The figure shows three views and two pictorial views of one solid part (mm, origin at its lowest corner). Answer the questions. A direction names the side the tool comes from. Give positions to 0.01 mm unless a question says otherwise; leave off trailing zeros. Write each loop counter-clockwise with the first axis right and the second up, starting at its lowest first coordinate (ties: lowest second). Pieces come first, ordered by that corner, then holes. Notation, with made-up numbers: M 36.5,7.25 L 87.5,7.25 A18 cw 87.5,22.25 Z; hole C 41,-24.5 d10. An arc over 180 degrees is marked long. Return JSON: item names as keys, results as strings.
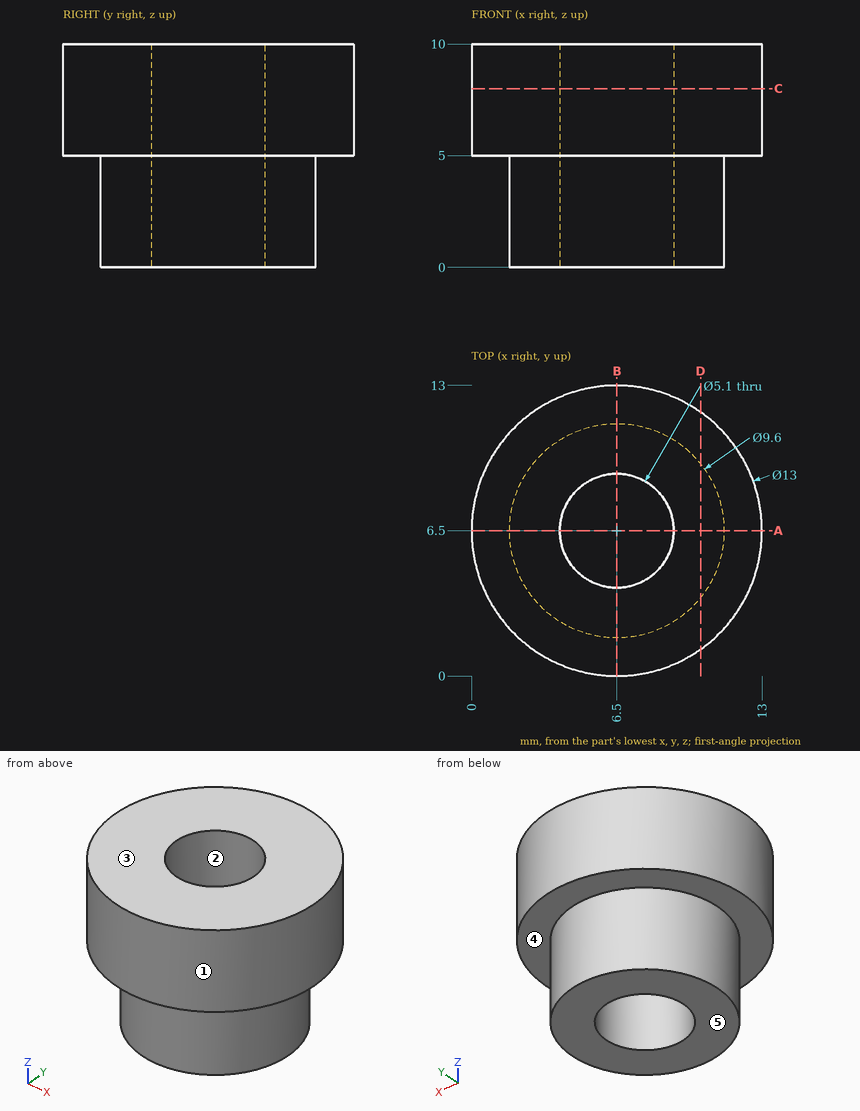
Item 1: Determine the mould class of the marked faces 1, 2 and 3 for opening direction X: +X half, -X half, draft (parallel to the pull), parting line (faces both ways), or undercut.
Geometry results:
{"face 1": "parting line", "face 2": "undercut", "face 3": "draft"}
Item 2: Given pin 1 Ø3 at (y, z) = (10.5, 1.5) entering from -X; pin 2 Ø2 at (x, z) = (9, 8) entering from +Y; pin 3 Ø1 at (y, z) = (11, 2) entering from -X, each flat-ended and moving along its own axis, determine where each tip first touches the part or whether it passes through.
Geometry results:
{"pin 1": "stops at x = 2.4", "pin 2": "stops at y = 12.82", "pin 3": "stops at x = 3.85"}
Item 3: A cutting plane is placed at A-A, the plane y = 6.5. Write down the section's boundary in (x, z), plus the area to 3 significant figures.
Geometry results:
{"outline": "M 0,5 L 1.7,5 L 1.7,0 L 3.95,0 L 3.95,10 L 0,10 Z; M 9.05,0 L 11.3,0 L 11.3,5 L 13,5 L 13,10 L 9.05,10 Z", "area": "62.0 mm2"}
Item 4: A cutting plane is placed at C-C, the plane z = 8. Write down the section's boundary in (x, y), plus the area to 3 significant figures.
Geometry results:
{"outline": "C 6.5,6.5 d13; hole C 6.5,6.5 d5.1", "area": "112 mm2"}
Item 5: A cutting plane is placed at D-D, the plane x = 10.25. Write down the section's boundary in (y, z), plus the area to 3 significant figures.
Geometry results:
{"outline": "M 1.19,5 L 3.5,5 L 3.5,0 L 9.5,0 L 9.5,5 L 11.81,5 L 11.81,10 L 1.19,10 Z", "area": "83.1 mm2"}
Item 6: Find the intervals of material crossed by line 1 (Y direction, x = 6.5, z = 4); line 2 (Y direction, x = 6.5, z = 6.5); line 3 (X direction, y = 5.5, z = 2.25), in increasing order.
Geometry results:
{"line 1": "y = 1.7 to 3.95, 9.05 to 11.3", "line 2": "y = 0 to 3.95, 9.05 to 13", "line 3": "x = 1.81 to 4.15, 8.85 to 11.19"}
Item 7: Which of the six approach directions +Z, -Z, +X, -X, +Y, -Y give full straight-line access (tool end or side, diameter ignored) to the marked faces 4 and 5?
Geometry results:
{"face 4": "-Z", "face 5": "-Z, +X, -X, +Y, -Y"}
